CAD build for the part. Positions are in the model's coordinates, mm. A direction names the side the tool comes from. Give positions to 0.01 mm unless a question says otherwise; leave off trailing zeros. Write each loop counter-clockwise with the first axis right and the second up, starting at its lowest first coordinate (ties: lowest second). Pieces come first, ordered by that corner, then holes. Notation, with made-up numbers: (11.5, -16) -> (37.5, -16) arc R36 cw to (37.5, 20) -> close; hole circle Ø5 at (-35.5, 15.5). An arc over 180 degrees is marked (long way). Answer in a Markdown table with one row per item. Add a question column.
```python
from build123d import *

# Parameters (mm, degrees)
F0_W     = 200.35
F0_H     = 146.35
F1_DEPTH = 5
F2_R     = 5
F3_W     = 189.9
F3_H     = 135.9
F4_DEPTH = 42.55
F5_R     = 3
F6_W     = 150
F6_H     = 100
F7_DEPTH = 1


with BuildPart() as f1:
    # F0 (on Front) → F1 (new body)
    with BuildSketch(Plane.XZ):
        Rectangle(F0_W, F0_H)
    extrude(amount=F1_DEPTH)

    # F2
    f2_edges = [f1.edges().sort_by_distance(p)[0] for p in [
        (100.175, -2.5, 73.175),
        (-100.175, -2.5, 73.175),
        (-100.175, -2.5, -73.175),
        (100.175, -2.5, -73.175),
    ]]
    fillet(f2_edges, radius=F2_R)

    # F3 (on face) → F4 (join)
    with BuildSketch(Plane(origin=(0, 0, 0), x_dir=(-1, 0, 0), z_dir=(0, 1, 0))):
        Rectangle(F3_W, F3_H)
    extrude(amount=-F4_DEPTH)

    # F5
    f5_edges = [f1.edges().sort_by_distance(p)[0] for p in [
        (100.175, 0, 0),
        (98.710534, 0, 71.710534),
        (0, 0, 73.175),
        (-98.710534, 0, 71.710534),
        (-100.175, 0, 0),
        (-98.710534, 0, -71.710534),
        (0, 0, -73.175),
        (98.710534, 0, -71.710534),
    ]]
    fillet(f5_edges, radius=F5_R)

    # F6 (on face) → F7 (cut)
    with BuildSketch(Plane(origin=(0, 0, 0), x_dir=(-1, 0, 0), z_dir=(0, 1, 0))):
        Rectangle(F6_W, F6_H)
    extrude(amount=-F7_DEPTH, mode=Mode.SUBTRACT)


solid = f1.part
```
Item 1: Slice it at C-C, the plane y = -17.5. List the corners of the cut face in (x, z).
Item 2: Drop flat-ended pins along their axis: pin 1 Ø5 at (x, y) = (1, -37) entering from -Z; pin 2 Ø0.8 at (y, z) = (-0.5, -14) entering from -X; pin 3 Ø0.5 at (x, y) = (32, -0.5) entering from +Z. Give the stop position or say it passes through.
Item 3: Slice it at B-B, the plane x = 9. List the corners of the cut face in (y, z) (3 decimals), then the cut area to 3 significant figures.
Item 4: Slice it at D-D, the plane x = 80. List the corners of the cut face in (y, z) (3 decimals).
Item 5: Probe L1, parallel to Z at x = 36.5, y = -16; L2, parallel to Y at x = -65.5, z = 6.5; L3, parallel to X at y = -8.5, z = -65.5. List the from-to ranges inside material, lowest first. Write a range as from..to.
Item 6: Mould opens along X. For faces 1 (the face through (98.75, -4.01, 71.67)), 2 (the face through (1, -1, 1)), 3 (the face through (-98.75, -4.01, -71.67)) say: released by +X, released by -X, zero draft, split by the parting line, or undercut.
Item 7: Slice it at A-A, the plane z = 56. List the corners of the cut face in (x, y) (3 decimals).
Item 8: Which spindle directions (+Z, -Z, +X, -X, +Y, -Y) get a long thin tool onto all of the face, cutting with end or side? Do faces 4 (the face through (-94.95, -24, -1)), 5 (the face through (1, -24, -67.95)), 6 (the face through (94.95, -24, -1)). Say none if no direction does.
Answer key:
| question | item | result |
|---|---|---|
| 1 | outline | (-94.95, -67.95) -> (94.95, -67.95) -> (94.95, 67.95) -> (-94.95, 67.95) -> close |
| 2 | pin 1 | stops at z = -67.95 |
| 2 | pin 2 | stops at x = -99.32 |
| 2 | pin 3 | stops at z = 72.16 |
| 3 | outline | (-42.55, -67.95) -> (-5, -67.95) -> (-5, -73.175) -> (-3, -73.175) arc R3 ccw to (0, -70.175) -> (0, -50) -> (-1, -50) -> (-1, 50) -> (0, 50) -> (0, 70.175) arc R3 ccw to (-3, 73.175) -> (-5, 73.175) -> (-5, 67.95) -> (-42.55, 67.95) -> close |
| 3 | area | 5,730 mm² |
| 4 | outline | (-42.55, -67.95) -> (-5, -67.95) -> (-5, -73.175) -> (-3, -73.175) arc R3 ccw to (0, -70.175) -> (0, 70.175) arc R3 ccw to (-3, 73.175) -> (-5, 73.175) -> (-5, 67.95) -> (-42.55, 67.95) -> close |
| 5 | L1 | z = -67.95..67.95 |
| 5 | L2 | y = -42.55..-1 |
| 5 | L3 | x = -94.95..94.95 |
| 6 | face 1 | released by +X |
| 6 | face 2 | undercut |
| 6 | face 3 | released by -X |
| 7 | outline | (-100.175, -5) -> (-94.95, -5) -> (-94.95, -42.55) -> (94.95, -42.55) -> (94.95, -5) -> (100.175, -5) -> (100.175, -3) arc R3 ccw to (97.175, 0) -> (-97.175, 0) arc R3 ccw to (-100.175, -3) -> close |
| 8 | face 4 | +Z, -Z, -X, -Y |
| 8 | face 5 | -Z, +X, -X, -Y |
| 8 | face 6 | +Z, -Z, +X, -Y |
